Check sheet for the modelled part. Datum: model origin and axes. Units: mm. Give positions to 0.01 mm unless a question says otherwise; leave off trailing zeros. Write each loop counter-clockwise with the first axis right and the second up, starting at its lowest first coordinate (ties: lowest second). Pieces come first, ordered by that corner, then holes. Notation, with made-up numbers: (-25, -7) -> (29, -7) arc R14 ccw to (29, 14) -> close; hole circle Ø5 at (63.25, 57.25). An arc over 180 degrees is marked (long way). Return JSON: item names as keys, results as strings.
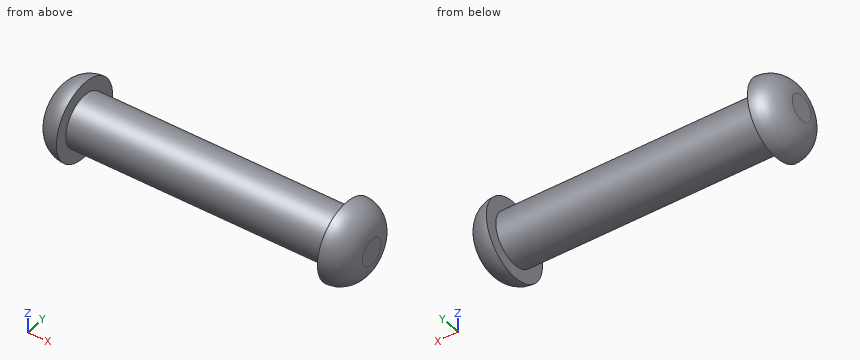
from build123d import *

# Parameters (mm, degrees)
FILLET1_R = 1


with BuildPart() as part:
    # Sketch2 → Revolve1 (revolve)
    with BuildSketch(Plane.XY, mode=Mode.PRIVATE) as revolve1_sk:
        Polygon((1, 1), (11, 1), (11, 1.5), (12, 1.5), (12, 0), (0, 0), (0, 1.5), (1, 1.5), align=None)
    revolve(revolve1_sk.sketch.rotate(Axis((12, 0, 0), (-1, 0, 0)), 90), axis=Axis((12, 0, 0), (-1, 0, 0)))

    # Fillet1
    fillet1_edges = [part.edges().sort_by_distance(p)[0] for p in [
        (0, 0, 1.5),
        (12, 0, 1.5),
    ]]
    fillet(fillet1_edges, radius=FILLET1_R - 0.0001)  # a hair under: the kernel refuses the full size


solid = part.part
(1) Thickness scan on L1, parallel to X at y = -0.55, z = -0.05; L2, parallel to Z at x = 9, y = -0.05; L3, parallel to X at y = -0.05, z = -1.25. Record the ranges inside material, lowest first.
Reply:
{"L1": "0 to 12", "L2": "-1 to 1", "L3": "0.34 to 1, 11 to 11.66"}
(2) Depth check by flat-ended pin: pin 1 Ø1 at (y, z) = (0.5, -1) entering from -X. Enter the tip coordinate at first touch or a pass-through.
Reply:
{"pin 1": "x = 0.01"}
(3) Cross-section at A-A on x = 1.25. Enter the section's corners in (y, z), then the cut area to 3 significant figures.
Reply:
{"outline": "circle Ø2 at (0, 0)", "area": "3.14 mm^2"}
